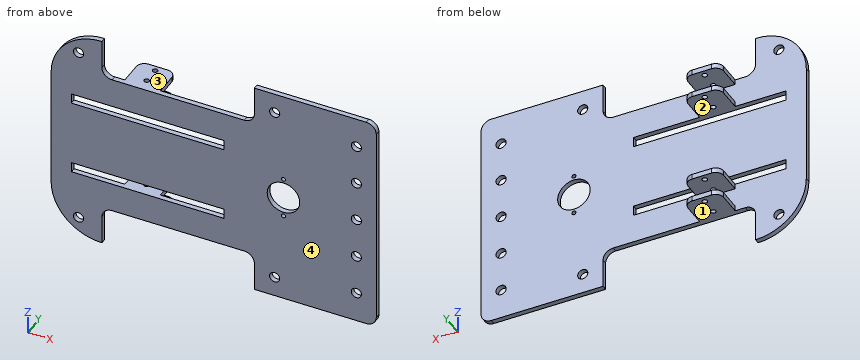
from build123d import *

# Parameters (mm, degrees)
SKETCH1_W           = 320
SKETCH1_H           = 220
BOSS_EXTRUDE1_DEPTH = 2.5
SKETCH2_R           = 5
CUT_EXTRUDE1_DEPTH  = 2.5
FILLET5_R           = 50
SKETCH3_W           = 150
SKETCH3_H           = 38.497712582
CUT_EXTRUDE2_DEPTH  = 2.5
FILLET3_R           = 10
SKETCH4_R           = 16
SKETCH4_R_2         = 2
CUT_EXTRUDE3_DEPTH  = 2.5
SKETCH6_R           = 5
CUT_EXTRUDE4_DEPTH  = 2.5
LPATTERN1_COUNT     = 3
LPATTERN1_PITCH     = 40
LPATTERN2_COUNT     = 3
LPATTERN2_PITCH     = 40
SKETCH8_W           = 35
SKETCH8_H           = 5
BOSS_EXTRUDE2_DEPTH = 30
CUT_EXTRUDE5_START  = -143.004575
SKETCH9_R           = 2.5
CUT_EXTRUDE5_DEPTH  = 143.004575
FILLET6_R           = 8
SKETCH10_W          = 150
SKETCH10_H          = 10
CUT_EXTRUDE6_DEPTH  = 33.75
FILLET7_R           = 10


with BuildPart() as part:
    # Sketch1 → Boss-Extrude1 (new, symmetric)
    with BuildSketch(Plane(origin=(0, 0, 0), x_dir=(1, 0, 0), z_dir=(0, 1, 0))):
        Rectangle(SKETCH1_W, SKETCH1_H)
    extrude(amount=BOSS_EXTRUDE1_DEPTH, both=True)

    # Sketch2 → Cut-Extrude1 (cut, symmetric)
    with BuildSketch(Plane(origin=(0, 0, 0), x_dir=(1, 0, 0), z_dir=(0, 1, 0))):
        with Locations(Location((-133, 90, 0), (0, 0, 270))):
            Circle(SKETCH2_R)
        with Locations(Location((-133, -90, 0), (0, 0, 270))):
            Circle(SKETCH2_R)
        with Locations(Location((60, 90, 0), (0, 0, 90))):
            Circle(SKETCH2_R)
        with Locations(Location((60, -90, 0), (0, 0, 90))):
            Circle(SKETCH2_R)
    extrude(amount=CUT_EXTRUDE1_DEPTH, both=True, mode=Mode.SUBTRACT)

    # Fillet5
    fillet5_edges = [part.edges().sort_by_distance(p)[0] for p in [
        (-160, 0, 110),
        (-160, 0, -110),
    ]]
    fillet(fillet5_edges, radius=FILLET5_R)

    # Sketch3 → Cut-Extrude2 (cut, symmetric)
    with BuildSketch(Plane(origin=(0, 0, 0), x_dir=(1, 0, 0), z_dir=(0, 1, 0))):
        with Locations((-35, 90.751143709)):
            Rectangle(SKETCH3_W, SKETCH3_H)
        with Locations((-35, -90.751143709)):
            Rectangle(SKETCH3_W, SKETCH3_H)
    extrude(amount=CUT_EXTRUDE2_DEPTH, both=True, mode=Mode.SUBTRACT)

    # Fillet3
    fillet3_edges = [part.edges().sort_by_distance(p)[0] for p in [
        (40, 0, -71.502287418),
        (-110, 0, -71.502287418),
        (-110, 0, 71.502287418),
        (40, 0, 71.502287418),
    ]]
    fillet(fillet3_edges, radius=FILLET3_R)

    # Sketch4 → Cut-Extrude3 (cut, symmetric)
    with BuildSketch(Plane(origin=(0, 0, 0), x_dir=(1, 0, 0), z_dir=(0, 1, 0))):
        with Locations(Location((68.657368821, 0, 0), (0, 0, 270))):
            Circle(SKETCH4_R)
        with Locations(Location((68.657368821, 20, 0), (0, 0, 270))):
            Circle(SKETCH4_R_2)
        with Locations(Location((68.657368821, -20, 0), (0, 0, 270))):
            Circle(SKETCH4_R_2)
    extrude(amount=CUT_EXTRUDE3_DEPTH, both=True, mode=Mode.SUBTRACT)

    # Sketch6 → Cut-Extrude4 (cut, symmetric)
    with BuildSketch(Plane(origin=(0, 0, 0), x_dir=(1, 0, 0), z_dir=(0, 1, 0))):
        with Locations(Location((140.361166029, 0, 0), (0, 0, 270))):
            Circle(SKETCH6_R)
    cut_extrude4 = extrude(amount=CUT_EXTRUDE4_DEPTH, both=True, mode=Mode.SUBTRACT)

    # LPattern1: Cut-Extrude4 ×3
    with Locations(*[(0, 0, -i * LPATTERN1_PITCH) for i in range(1, LPATTERN1_COUNT)]):
        add(cut_extrude4, mode=Mode.SUBTRACT)

    # LPattern2: Cut-Extrude4 ×3
    with Locations(*[(0, 0, i * LPATTERN2_PITCH) for i in range(1, LPATTERN2_COUNT)]):
        add(cut_extrude4, mode=Mode.SUBTRACT)

    # Sketch8 → Boss-Extrude2 (add)
    with BuildSketch(Plane(origin=(0, 2.5, 0), x_dir=(1, 0, 0), z_dir=(0, 1, 0))):
        with Locations((-72.5, -69.002287418)):
            Rectangle(SKETCH8_W, SKETCH8_H)
        with Locations((-72.5, -45.002287418)):
            Rectangle(SKETCH8_W, SKETCH8_H)
        with Locations((-72.5, 45.002287418)):
            Rectangle(SKETCH8_W, SKETCH8_H)
        with Locations((-72.5, 69.002287418)):
            Rectangle(SKETCH8_W, SKETCH8_H)
    extrude(amount=BOSS_EXTRUDE2_DEPTH)

    # Sketch9 → Cut-Extrude5 (cut)
    with BuildSketch(Plane.XY.offset(71.502287418).offset(CUT_EXTRUDE5_START)):
        with Locations((-72.5, 26.744818561)):
            Circle(SKETCH9_R)
        with Locations((-72.5, 10.250757787)):
            Circle(SKETCH9_R)
    extrude(amount=CUT_EXTRUDE5_DEPTH, mode=Mode.SUBTRACT)

    # Fillet6
    fillet6_edges = [part.edges().sort_by_distance(p)[0] for p in [
        (-90, 32.5, 69.002287418),
        (-55, 32.5, 69.002287418),
        (-90, 32.5, 45.002287418),
        (-55, 32.5, 45.002287418),
        (-90, 32.5, -45.002287418),
        (-55, 32.5, -45.002287418),
        (-90, 32.5, -69.002287418),
        (-55, 32.5, -69.002287418),
    ]]
    fillet(fillet6_edges, radius=FILLET6_R)

    # Sketch10 → Cut-Extrude6 (cut, symmetric)
    with BuildSketch(Plane(origin=(0, 0, 0), x_dir=(1, 0, 0), z_dir=(0, 1, 0))):
        with Locations((-65, -37.502287418)):
            Rectangle(SKETCH10_W, SKETCH10_H)
        with Locations((-65, 37.502287418)):
            Rectangle(SKETCH10_W, SKETCH10_H)
    extrude(amount=CUT_EXTRUDE6_DEPTH, both=True, mode=Mode.SUBTRACT)

    # Fillet7
    fillet7_edges = [part.edges().sort_by_distance(p)[0] for p in [
        (160, 0, 110),
        (160, 0, -110),
    ]]
    fillet(fillet7_edges, radius=FILLET7_R)


solid = part.part
Can you work these out from the model? Positions are in its coordinate system, mm. Face numbers are marked on the shaded views. Give positions to 0.01 mm unless a question says otherwise; leave off trailing zeros. Loops run counter-clockwise (first coordinate to the right, second up) from the corner with the lowest first, then second, coordinate; pieces in that order, holes last. Notation, with made-up numbers: (36, 72) - (48, 72) arc R17 ccw to (48, 85) - close; hole circle Ø4 at (15, 45). An arc over 180 degrees is marked (long way). Return JSON: item names as keys, results as strings.
1. I want a section at B-B on x = -22.5. Please give me the cut outline in (y, z).
Output values:
{"outline": "(-2.5, -71.5) - (2.5, -71.5) - (2.5, -42.5) - (-2.5, -42.5) - close; (-2.5, -32.5) - (2.5, -32.5) - (2.5, 32.5) - (-2.5, 32.5) - close; (-2.5, 42.5) - (2.5, 42.5) - (2.5, 71.5) - (-2.5, 71.5) - close"}
2. We'd pull the mould along Z, two halves only. Please class the marked faces 1, 2, 3 and 4: +Z half, -Z half, draft (parallel to the pull), parting line (faces both ways), or undercut.
Output values:
{"face 1": "-Z half", "face 2": "undercut", "face 3": "+Z half", "face 4": "draft"}
3. I'm going to push flat-ended pins straight in: pin 1 Ø15 at (x, y) = (-64, 13) entering from -Z; pin 2 Ø12 at (y, z) = (28.5, 43.5) entering from +X; pin 3 Ø8 at (x, z) = (31, -19) entering from +Y. Where does each tip first touch, or does it pass through?
Output values:
{"pin 1": "stops at z = -71.5", "pin 2": "stops at x = -55", "pin 3": "stops at y = 2.5"}
4. If I drill on line 1 (Y direction, x = -72, z = -43); line 2 (Z direction, x = -79.5, y = 14); line 3 (X direction, y = 0, z = 0), over which ranges is the centre line in solid material (lowest first)?
Output values:
{"line 1": "y = -2.5 to 7.8, 12.7 to 24.3, 29.19 to 32.5", "line 2": "z = -71.5 to -66.5, -47.5 to -42.5, 42.5 to 47.5, 66.5 to 71.5", "line 3": "x = -160 to 52.66, 84.66 to 135.36, 145.36 to 160"}
5. I want a section at A-A on z = 90. Please give me the cut outline in (x, y).
Output values:
{"outline": "(-150, -2.5) - (-138, -2.5) - (-138, 2.5) - (-150, 2.5) - close; (-128, -2.5) - (-110, -2.5) - (-110, 2.5) - (-128, 2.5) - close; (40, -2.5) - (55, -2.5) - (55, 2.5) - (40, 2.5) - close; (65, -2.5) - (160, -2.5) - (160, 2.5) - (65, 2.5) - close"}
6. I want a section at D-D on x = 18. Please give me the cut outline in (y, z).
Output values:
{"outline": "(-2.5, -71.5) - (2.5, -71.5) - (2.5, 71.5) - (-2.5, 71.5) - close"}
7. I want a section at C-C on x = -133. Please give me the cut outline in (y, z).
Output values:
{"outline": "(-2.5, -104.4) - (2.5, -104.4) - (2.5, -95) - (-2.5, -95) - close; (-2.5, -85) - (2.5, -85) - (2.5, -42.5) - (-2.5, -42.5) - close; (-2.5, -32.5) - (2.5, -32.5) - (2.5, 32.5) - (-2.5, 32.5) - close; (-2.5, 42.5) - (2.5, 42.5) - (2.5, 85) - (-2.5, 85) - close; (-2.5, 95) - (2.5, 95) - (2.5, 104.4) - (-2.5, 104.4) - close"}
